Verification items for the finished model (mm, model axes). A direction names the side the tool comes from. Give positions to 0.01 mm unless a question says otherwise; leave off trailing zeros. Loops run counter-clockwise (first coordinate to the right, second up) from the corner with the lowest first, then second, coordinate; pieces in that order, holes last. Notation, with made-up numbers: M 82.25,-25 L 124.25,-25 A21 cw 124.25,2 Z; hole C 38.25,64.5 d8. An arc over 180 degrees is marked long. Answer in a Markdown table with one row per item.
```python
from build123d import *

# Parameters (mm, degrees)
F0_W      = 320
F0_H      = 420
F1_DEPTH  = 4
F3_DEPTH  = 4
F4_R      = 3
F5_DEPTH  = 25
F6_R      = 3
F7_DEPTH  = 25
F8_R      = 3
F9_DEPTH  = 25
F11_DEPTH = 25
F13_DEPTH = 25


with BuildPart() as f1:
    # F0 (on Top) → F1 (new body)
    with BuildSketch(Plane.XY):
        with Locations((160, 210)):
            Rectangle(F0_W, F0_H)
    extrude(amount=F1_DEPTH)

    # F2 (on face) → F3 (cut, through all)
    with BuildSketch(Plane.XY.offset(4)):
        Polygon((320, 420), (290, 420), (320, 360), align=None)
        Polygon((320, 60), (290, 0), (320, 0), align=None)
        with BuildLine():
            Line((113, 360), (213, 360))
            ThreePointArc((213, 360), (216.535534, 361.464466), (218, 365))
            Line((218, 365), (218, 403))
            ThreePointArc((218, 403), (216.535534, 406.535534), (213, 408))
            Line((213, 408), (113, 408))
            ThreePointArc((113, 408), (109.464466, 406.535534), (108, 403))
            Line((108, 403), (108, 365))
            ThreePointArc((108, 365), (109.464466, 361.464466), (113, 360))
        make_face()
        with BuildLine():
            Line((113, 12), (213, 12))
            ThreePointArc((213, 12), (216.535534, 13.464466), (218, 17))
            Line((218, 17), (218, 55))
            ThreePointArc((218, 55), (216.535534, 58.535534), (213, 60))
            Line((213, 60), (113, 60))
            ThreePointArc((113, 60), (109.464466, 58.535534), (108, 55))
            Line((108, 55), (108, 17))
            ThreePointArc((108, 17), (109.464466, 13.464466), (113, 12))
        make_face()
        Polygon((0, 420), (0, 210), (50, 420), align=None)
        Polygon((50, 0), (0, 210), (0, 0), align=None)
    extrude(amount=-F3_DEPTH, mode=Mode.SUBTRACT)

    # F4 (on face) → F5 (cut)
    with BuildSketch(Plane.XY.offset(4)):
        with Locations((67, 6)):
            Circle(F4_R)
        with Locations((97, 6)):
            Circle(F4_R)
        with Locations((127, 6)):
            Circle(F4_R)
        with Locations((157, 6)):
            Circle(F4_R)
        with Locations((187, 6)):
            Circle(F4_R)
        with Locations((217, 6)):
            Circle(F4_R)
        with Locations((247, 6)):
            Circle(F4_R)
        with Locations((277, 6)):
            Circle(F4_R)
        with Locations((64, 66)):
            Circle(F4_R)
        with Locations((94, 66)):
            Circle(F4_R)
        with Locations((124, 66)):
            Circle(F4_R)
        with Locations((220, 66)):
            Circle(F4_R)
        with Locations((250, 66)):
            Circle(F4_R)
        with Locations((280, 66)):
            Circle(F4_R)
        with Locations((310, 66)):
            Circle(F4_R)
        with Locations((67, 414)):
            Circle(F4_R)
        with Locations((64, 354)):
            Circle(F4_R)
        with Locations((97, 414)):
            Circle(F4_R)
        with Locations((310, 354)):
            Circle(F4_R)
        with Locations((277, 414)):
            Circle(F4_R)
        with Locations((94, 354)):
            Circle(F4_R)
        with Locations((220, 354)):
            Circle(F4_R)
        with Locations((280, 354)):
            Circle(F4_R)
        with Locations((124, 354)):
            Circle(F4_R)
        with Locations((127, 414)):
            Circle(F4_R)
        with Locations((250, 354)):
            Circle(F4_R)
        with Locations((157, 414)):
            Circle(F4_R)
        with Locations((187, 414)):
            Circle(F4_R)
        with Locations((217, 414)):
            Circle(F4_R)
        with Locations((247, 414)):
            Circle(F4_R)
    extrude(amount=-F5_DEPTH, mode=Mode.SUBTRACT)

    # F6 (on face) → F7 (cut)
    with BuildSketch(Plane.XY.offset(4)):
        with Locations((121, 90)):
            Circle(F6_R)
        with Locations((121, 130)):
            Circle(F6_R)
        with Locations((121, 170)):
            Circle(F6_R)
        with Locations((206, 90)):
            Circle(F6_R)
        with Locations((206, 130)):
            Circle(F6_R)
        with Locations((206, 170)):
            Circle(F6_R)
        with Locations((291, 80)):
            Circle(F6_R)
        with Locations((291, 120)):
            Circle(F6_R)
        with Locations((291, 160)):
            Circle(F6_R)
        with Locations((121, 330)):
            Circle(F6_R)
        with Locations((121, 290)):
            Circle(F6_R)
        with Locations((206, 330)):
            Circle(F6_R)
        with Locations((206, 250)):
            Circle(F6_R)
        with Locations((291, 340)):
            Circle(F6_R)
        with Locations((121, 250)):
            Circle(F6_R)
        with Locations((206, 290)):
            Circle(F6_R)
        with Locations((291, 300)):
            Circle(F6_R)
        with Locations((291, 260)):
            Circle(F6_R)
    extrude(amount=-F7_DEPTH, mode=Mode.SUBTRACT)

    # F8 (on face) → F9 (cut)
    with BuildSketch(Plane.XY.offset(4)):
        with Locations((15, 210)):
            Circle(F8_R)
        with Locations((45, 210)):
            Circle(F8_R)
    extrude(amount=-F9_DEPTH, mode=Mode.SUBTRACT)

    # F10 (on face) → F11 (intersect)
    with BuildSketch(Plane.XY.offset(4)):
        with BuildLine():
            Line((87, 350), (87, 355))
            ThreePointArc((87, 355), (85.535534, 358.535534), (82, 360))
            Line((82, 360), (57, 360))
            ThreePointArc((57, 360), (53.464466, 358.535534), (52, 355))
            Line((52, 355), (52, 340))
            ThreePointArc((52, 340), (50.535534, 336.464466), (47, 335))
            Line((47, 335), (0, 335))
            Line((0, 335), (0, 210))
            Line((0, 210), (0, 85))
            Line((0, 85), (47, 85))
            ThreePointArc((47, 85), (50.535534, 83.535534), (52, 80))
            Line((52, 80), (52, 65))
            ThreePointArc((52, 65), (53.464466, 61.464466), (57, 60))
            Line((57, 60), (82, 60))
            ThreePointArc((82, 60), (85.535534, 61.464466), (87, 65))
            Line((87, 65), (87, 70))
            ThreePointArc((87, 70), (88.464466, 73.535534), (92, 75))
            Line((92, 75), (275, 75))
            ThreePointArc((275, 75), (278.535534, 76.464466), (280, 80))
            Line((280, 80), (280, 82))
            ThreePointArc((280, 82), (281.464466, 85.535534), (285, 87))
            Line((285, 87), (320, 87))
            Line((320, 87), (320, 210))
            Line((320, 210), (320, 333))
            Line((320, 333), (285, 333))
            ThreePointArc((285, 333), (281.464466, 334.464466), (280, 338))
            Line((280, 338), (280, 340))
            ThreePointArc((280, 340), (278.535534, 343.535534), (275, 345))
            Line((275, 345), (92, 345))
            ThreePointArc((92, 345), (88.464466, 346.464466), (87, 350))
        make_face()
    extrude(amount=-F11_DEPTH, mode=Mode.INTERSECT)

    # F12 (on face) → F13 (intersect)
    with BuildSketch(Plane.XY.offset(4)):
        with BuildLine():
            Line((320, 75), (320, 345))
            Line((320, 345), (200, 345))
            Line((200, 345), (200, 265))
            ThreePointArc((200, 265), (201.464466, 261.464466), (205, 260))
            Line((205, 260), (210, 260))
            ThreePointArc((210, 260), (213.535534, 258.535534), (215, 255))
            Line((215, 255), (215, 165))
            ThreePointArc((215, 165), (213.535534, 161.464466), (210, 160))
            Line((210, 160), (205, 160))
            ThreePointArc((205, 160), (201.464466, 158.535534), (200, 155))
            Line((200, 155), (200, 75))
            Line((200, 75), (320, 75))
        make_face()
    extrude(amount=-F13_DEPTH, mode=Mode.INTERSECT)


solid = f1.part
```
Item 1: Sectioned sample at A-A (y = 120). Record the cut outline in (x, z).
Reported:
| item | result |
|---|---|
| outline | M 200,0 L 288,0 L 288,4 L 200,4 Z; M 294,0 L 320,0 L 320,4 L 294,4 Z |
Item 2: Sectioned sample at C-C (z = 1.55). State how many separate pieces and enclosed holes the cut face has, and give its area (3 significant figures).
Reported:
| item | result |
|---|---|
| separate pieces | 1 |
| enclosed holes | 8 |
| area | 29,700 mm^2 |
Item 3: Sectioned sample at B-B (x = 291). Record the cut outline in (y, z), and give its area (3 significant figures).
Reported:
| item | result |
|---|---|
| outline | M 87,0 L 117,0 L 117,4 L 87,4 Z; M 123,0 L 157,0 L 157,4 L 123,4 Z; M 163,0 L 257,0 L 257,4 L 163,4 Z; M 263,0 L 297,0 L 297,4 L 263,4 Z; M 303,0 L 333,0 L 333,4 L 303,4 Z |
| area | 888 mm^2 |
Item 4: Go/stop test with flat-tipped pins: pin 1 (9.5 mm diameter, centred on x = 206, y = 290, fed in from +Z); pin 2 (1 mm diameter, centred on x = 280, z = 2, fed in from -Y); pin 3 (3.5 mm diameter, centred on x = 291, y = 300, fed in from +Z); pin 4 (0.6 mm diameter, centred on y = 81, z = 1.5, fed in from +X). Record where each tip stops, or that it passes through.
Reported:
| item | result |
|---|---|
| pin 1 | stops at z = 4 |
| pin 2 | stops at y = 77.82 |
| pin 3 | passes through |
| pin 4 | stops at x = 280 |
Item 5: Scan lines: L1, parallel to Y at x = 291, z = 2.05; L2, parallel to Y at x = 206, z = 1.4; L3, parallel to X at y = 330, z = 1.15. Record each from-to range of solid material in increasing order. Write a range as [from, to].
Reported:
| item | result |
|---|---|
| L1 | y = [87, 117], [123, 157], [163, 257], [263, 297], [303, 333] |
| L2 | y = [75, 87], [93, 127], [133, 160], [260, 287], [293, 327], [333, 345] |
| L3 | x = [200, 203], [209, 320] |
Item 6: Sectioned sample at D-D (x = 212.5). Record the cut outline in (y, z), and give its area (3 significant figures).
Reported:
| item | result |
|---|---|
| outline | M 75,0 L 160.67,0 L 160.67,4 L 75,4 Z; M 259.33,0 L 345,0 L 345,4 L 259.33,4 Z |
| area | 685 mm^2 |
Item 7: Release check for a two-part mould opening along X. For faces 3 (the flat face through (259, 212, 0)), 4 (the cylindrical face through (281, 85, 2)), 5 (the cylindrical face through (288.79, 162.03, 2.03)) record: released by +X, released by -X, zero draft, split by the parting line, or undercut.
Reported:
| item | result |
|---|---|
| face 3 | zero draft |
| face 4 | released by +X |
| face 5 | undercut |
Item 8: Tool access check on faces 1 (the cylindrical face through (291, 303, 2)), 2 (the cylindrical face through (202, 159, 2)). Record the directions out of +Z, -Z, +X, -X, +Y, -Y that give a thin tool (end or side, any length) a straight path to the whole face; none if there is none.
Reported:
| item | result |
|---|---|
| face 1 | +Z, -Z |
| face 2 | +Z, -Z, -X |
